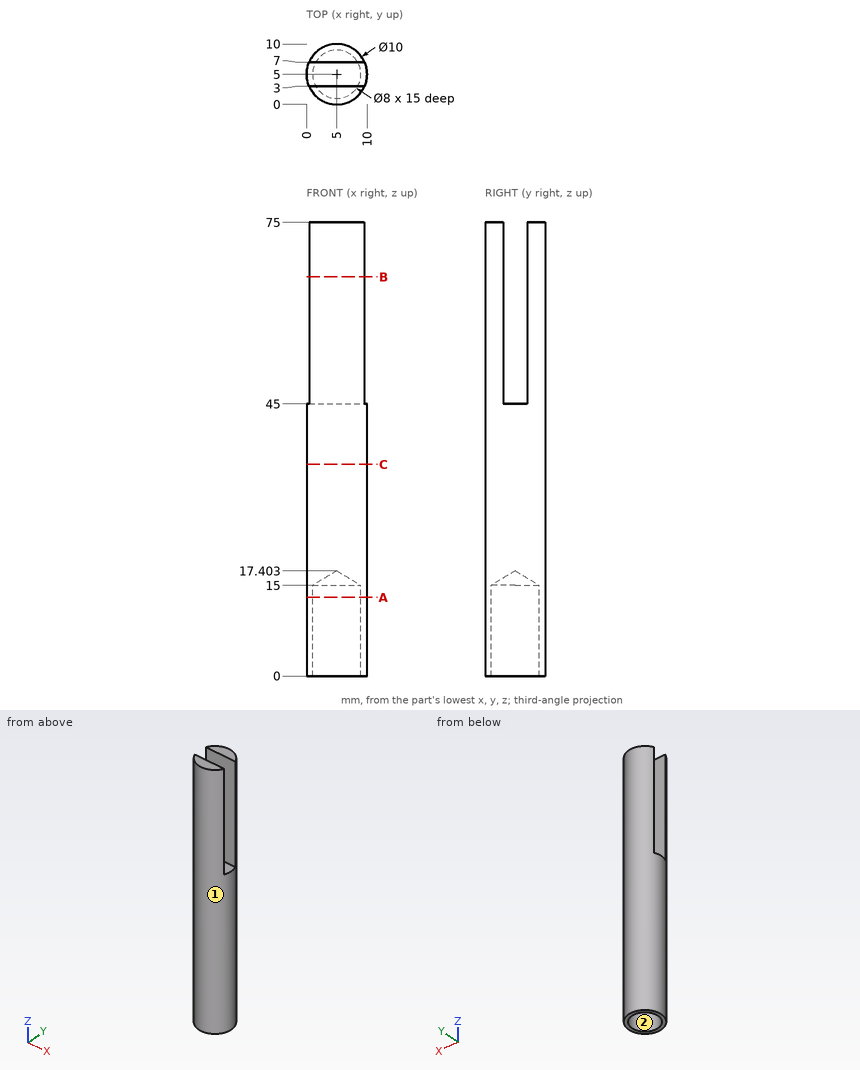
Check sheet for the drawn part. Datum: minimum x, y, z corner. Units: mm. Round coordinates to 2 decimals unless told otherwise and drop trailing zeros. Order: outer loops, then holes, each group sorted by start corner. A loop starts at its lowest first (then second) coordinate and runs counter-clockwise, first axis right, second up.
1. Thickness scan on L1, parallel to Y at x = 5, z = 11.5; L2, parallel to X at y = 8, z = 51; L3, parallel to Y at x = 8, z = 10 (1 decimal). Record the ranges inside material, lowest first.
Final values:
L1: y = 0 to 1, 9 to 10
L2: x = 1 to 9
L3: y = 1 to 2.4, 7.6 to 9
2. Section check A-A on z = 13. Record the cut outline in (x, y).
Final values:
outline: circle Ø10 at (5, 5); hole circle Ø8 at (5, 5)
3. Section check C-C on z = 35. Record the cut outline in (x, y).
Final values:
outline: circle Ø10 at (5, 5)
4. Go/stop test with flat-tipped pins: P1, Ø1, axis at x = 4, y = 6, coming from the -Z side; P2, Ø2.5, axis at x = 3.5, z = 66.5, coming from the +Y side; P3, Ø1.5, axis at y = 3, z = 40, coming from the -X side; P4, Ø4.5, axis at x = 3.5, z = 57.5, coming from the -Y side. Record where each tip stops, or that it passes through.
Final values:
P1: stops at z = 16.25
P2: stops at y = 9.99
P3: stops at x = 0.16
P4: stops at y = 0
5. Section check B-B on z = 66. Record the cut outline in (x, y).
Final values:
outline: (0.42, 3) arc R5 ccw to (9.58, 3) - close; (0.42, 7) - (9.58, 7) arc R5 ccw to start
6. Release check for a two-part mould opening along X. For the marked faces 1 and 2 record: +X half, -X half, draft (parallel to the pull), parting line (faces both ways), or undercut.
Final values:
face 1: parting line
face 2: undercut
